Input: part model. Units: mm. Frame: model coordinates. Round coordinates to 2 decimals unless told otherwise and drop trailing zeros. Loops run counter-clockwise (first coordinate to the right, second up) from the corner with the lowest first, then second, coordinate; pieces in that order, holes last. Notation, with made-up numbers: (-37, 8.5) -> (2, 8.5) arc R15 ccw to (2, 15.5) -> close; hole circle Ø7 at (67, 8.25). An arc over 180 degrees is marked (long way). Answer as a JSON object with one key per item and string values.
```python
from build123d import *

# Parameters (mm, degrees)
BOSS_EXTRUDE1_DEPTH = 1828.8
THRU_HOLES_D        = 2.794


with BuildPart() as part:
    # Sketch1 → Boss-Extrude1 (new body)
    with BuildSketch(Plane(origin=(0, 0, 0), x_dir=(1, 0, 0), z_dir=(0, 1, 0))):
        with BuildLine():
            Line((-3.048, 13.208), (-3.048, 4.953))
            ThreePointArc((-3.048, 4.953), (-3.085197439, 4.863197439), (-3.175, 4.826))
            Line((-3.175, 4.826), (-4.826, 4.826))
            ThreePointArc((-4.826, 4.826), (-5.005605122, 4.751605122), (-5.08, 4.572))
            Line((-5.08, 4.572), (-5.08, 0))
            ThreePointArc((-5.08, 0), (-3.592102448, -3.592102448), (0, -5.08))
            Line((0, -5.08), (4.572, -5.08))
            ThreePointArc((4.572, -5.08), (4.751605122, -5.005605122), (4.826, -4.826))
            Line((4.826, -4.826), (4.826, -3.175))
            ThreePointArc((4.826, -3.175), (4.863197439, -3.085197439), (4.953, -3.048))
            Line((4.953, -3.048), (13.208, -3.048))
            ThreePointArc((13.208, -3.048), (13.746815367, -2.824815367), (13.97, -2.286))
            Line((13.97, -2.286), (13.97, 7.304369265))
            ThreePointArc((13.97, 7.304369265), (13.911996204, 7.595974041), (13.746815367, 7.843184633))
            Line((13.746815367, 7.843184633), (7.843184633, 13.746815367))
            ThreePointArc((7.843184633, 13.746815367), (7.595974041, 13.911996204), (7.304369265, 13.97))
            Line((7.304369265, 13.97), (-2.286, 13.97))
            ThreePointArc((-2.286, 13.97), (-2.824815367, 13.746815367), (-3.048, 13.208))
        make_face()
    extrude(amount=BOSS_EXTRUDE1_DEPTH)

    # THRU HOLES (through all)
    with Locations(Plane(origin=(0, 1828.8, 0), x_dir=(1, 0, 0), z_dir=(0, 1, 0))):
        with Locations((0, 0), (2.54, 10.16), (10.16, 2.54)):
            Hole(THRU_HOLES_D / 2)


solid = part.part
```
1) Contact query for flat-ended pins moving along their axis: P1, Ø3, axis at x = 2.54, z = -10.16, coming from the +Y side; P2, Ø6.5, axis at x = 8.5, y = 826, coming from the +Z side; P3, Ø4, axis at y = 1097.5, z = -11, coming from the -X side; P4, Ø0.5, axis at x = -4, y = 795, coming from the -Z side. Output: stop coordinate, or through.
Output:
{"P1": "stops at y = 1828.8", "P2": "stops at z = 3.05", "P3": "stops at x = -3.05", "P4": "stops at z = -4.83"}
2) Ray query, probe 1 along Z at (x, y) = (2, 1018); probe 2 along X at (y, z) = (285, -3.25); probe 3 along Z at (x, y) = (10.16, 1452.5). Return the intervals inside material, ascending.
Output:
{"probe 1": "z = -13.97 to -11.45, -8.87 to 5.08", "probe 2": "x = -5.08 to 8.96, 11.36 to 13.97", "probe 3": "z = -11.43 to -3.94, -1.14 to 3.05"}
3) Section A-A, the plane y = 1091.5. Output: boundary loops of the cut face in (x, z) (3 decimals).
Output:
{"outline": "(-5.08, -4.572) arc R0.254 ccw to (-4.826, -4.826) -> (-3.175, -4.826) arc R0.127 cw to (-3.048, -4.953) -> (-3.048, -13.208) arc R0.762 ccw to (-2.286, -13.97) -> (7.304, -13.97) arc R0.762 ccw to (7.843, -13.747) -> (13.747, -7.843) arc R0.762 ccw to (13.97, -7.304) -> (13.97, 2.286) arc R0.762 ccw to (13.208, 3.048) -> (4.953, 3.048) arc R0.127 cw to (4.826, 3.175) -> (4.826, 4.826) arc R0.254 ccw to (4.572, 5.08) -> (0, 5.08) arc R5.08 ccw to (-5.08, 0) -> close; hole circle Ø2.794 at (0, 0); hole circle Ø2.794 at (2.54, -10.16); hole circle Ø2.794 at (10.16, -2.54)"}
